Part model, mm, in its own coordinate system. Face numbers are marked on the shaded views. A direction names the side the tool comes from. Round coordinates to 2 decimals unless told otherwise and drop trailing zeros. Loops run counter-clockwise (first coordinate to the right, second up) from the corner with the lowest first, then second, coordinate; pieces in that order, holes last. Notation, with made-up numbers: (-18.75, 45) - (39.25, 45) arc R29 ccw to (39.25, 66) - close; hole circle Ø9 at (40, 28.5). An arc over 180 degrees is marked (long way). Put each result on its own line as item: value.
Autodesk Inventor part; units mm, degrees
ref_plane "YZ Plane" through (0, 0, 0) normal (1, 0, 0) x (0, 1, 0)
ref_plane "XZ Plane" through (0, 0, 0) normal (0, 1, 0) x (-1, 0, 0)
ref_plane "XY Plane" through (0, 0, 0) normal (0, 0, 1) x (1, 0, 0)
sketch "Sketch1" plane through (0, 0, 0) normal (0, 0, 1) x (1, 0, 0)
  line L0 (0, 0) -> (-38.1, 0)
  line L1 (-19.05, 0) -> (-19.05, -38.1)
  line L2 (-19.05, -38.1) -> (-38.1, -38.1)
  line L3 (-38.1, -38.1) -> (-38.1, 0)
  line L4 (-19.05, -38.1) -> (0, -38.1)
  line L5 (0, 0) -> (0, -38.1)
  dimension "d0" = 38.1
  dimension "d1" = 38.1
  dimension "d2" = 19.05
  dimension "d3" = 19.05
extrude "Plate1" add sketch "Sketch1" along normal blind 3.048
sketch "Sketch2" plane through (0, 0, 3.048) normal (0, 0, 1) x (1, 0, 0)
  line L0 (-38.1, 0) -> (0, 0)
  line L1 (0, -38.1) -> (-38.1, -38.1)
  line L2 (-19.05, 0) -> (-19.05, -19.05)
  circle A0 centre (-19.05, -19.05) radius 14.2875
  dimension "d7" = 19.05
  dimension "d8" = 28.575
extrude "Cut1" cut sketch "Sketch2" against normal blind 3.048
sketch "Sketch3" plane through (-38.1, -41.148, -3.048) normal (0, -1, 0) x (1, 0, 0)
  line L0 (38.1, 0) -> (0, 0)
  line L1 (0, 0) -> (0, -19.304)
  line L2 (0, -19.304) -> (38.1, -19.304)
  line L3 (38.1, -19.304) -> (38.1, 0)
edge flange "Flange1" height 25.4 angle 90 thickness 3.048 bend radius 3.048 thickness toward (0, -1, 0) relief straight relief width 3.048 relief depth 1.524 edges at (-19.05, -38.1, 0) wall of the first edge with corners at (0, -41.148, -3.048) (-38.1, -41.148, -3.048) (-38.1, -41.148, -22.352) (0, -41.148, -22.352)
bend "Bend1"
corner "Corner1"
sketch "Sketch5" plane through (-38.1, -41.148, -22.352) normal (0, 1, 0) x (1, 0, 0)
  line L0 (0, -19.304) -> (38.1, -19.304)
  line L1 (38.1, 0) -> (38.1, -19.304)
  line L2 (38.1, 0) -> (0, 0)
  line L3 (0, 0) -> (0, -19.304)
  point P0 (38.1, -22.352)
equation "\"d9\" = Thickness"
equation "\"d11\" = BendReliefWidth"
equation "\"d12\" = BendReliefDepth"
equation "\"d13\" = MinimumRemnant"
equation "\"d14\" = BendRadius"
equation "\"d17\" = BendRadius"
equation "\"d18\" = CornerReliefSize"
equation "\"d19\" = GapSize"
equation "\"d20\" = JacobiRadiusSize"
equation "\"BendRadius\" = Thickness"
equation "\"BendReliefWidth\" = Thickness"
equation "\"BendReliefDepth\" = 0.5 * Thickness"
equation "\"CornerReliefSize\" = 4 * Thickness"
equation "\"MinimumRemnant\" = 2 * Thickness"
equation "\"TransitionRadius\" = BendRadius"
equation "\"JacobiRadiusSize\" = Thickness"
equation "\"GapSize\" = Thickness"
equation "\"d4\" = BendRadius"
properties part number "arm assembly outer mount"
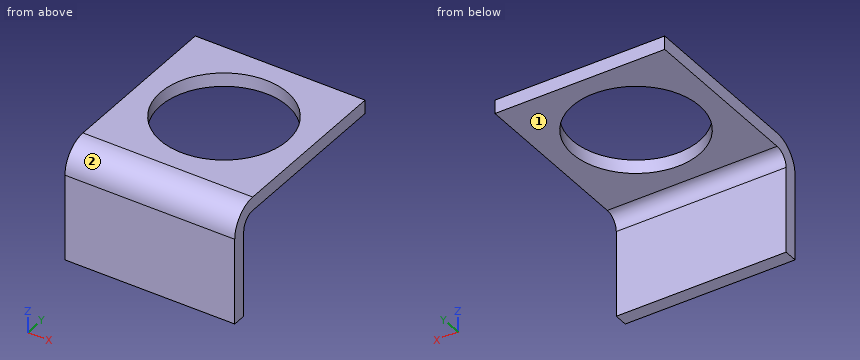
1. Band-saw the part on B-B (y = -19.05). List the corners of the cut face in (x, z), plus the area to 3 significant figures.
A:
outline: (-38.1, 0) - (-33.34, 0) - (-33.34, 3.05) - (-38.1, 3.05) - close; (-4.76, 0) - (0, 0) - (0, 3.05) - (-4.76, 3.05) - close
area: 29.0 mm²
2. Pin check, flat tip, straight feed: P1, Ø17, axis at x = -19.05, y = -19.05, coming from the -Z side. Stop position of the tip, or through.
A:
P1: passes through
3. Band-saw the part on D-D (x = -30.5). List the corners of the cut face in (y, z), plus the area to 3 significant figures.
A:
outline: (-44.2, -22.35) - (-41.15, -22.35) - (-41.15, -3.05) arc R3.05 cw to (-38.1, 0) - (-27.6, 0) - (-27.6, 3.05) - (-38.1, 3.05) arc R6.1 ccw to (-44.2, -3.05) - close; (-10.5, 0) - (0, 0) - (0, 3.05) - (-10.5, 3.05) - close
area: 145 mm²
4. Band-saw the part on A-A (x = -19.05). List the corners of the cut face in (y, z).
A:
outline: (-44.2, -22.35) - (-41.15, -22.35) - (-41.15, -3.05) arc R3.05 cw to (-38.1, 0) - (-33.34, 0) - (-33.34, 3.05) - (-38.1, 3.05) arc R6.1 ccw to (-44.2, -3.05) - close; (-4.76, 0) - (0, 0) - (0, 3.05) - (-4.76, 3.05) - close
5. Band-saw the part on C-C (z = -13.25). List the corners of the cut face in (x, y).
A:
outline: (-38.1, -44.2) - (0, -44.2) - (0, -41.15) - (-38.1, -41.15) - close
6. Tool access for the marked faces 1 and 2: list every direction of +Z, -Z, +X, -X, +Y, -Y with a clear straight run to the whole face (end or side of a thin tool).
A:
face 1: -Z, +X, -X, +Y
face 2: +Z, +X, -X, -Y
7. Probe line 1 along X through (y, z) = (-19.05, 0.95); line 2 along Y through (x, z) = (-1.5, -6.25); line 3 along Z through (x, y) = (-5, -10). List the from-to ranges inside material, lowest first. Write a range as [from, to].
A:
line 1: x = [-38.1, -33.34], [-4.76, 0]
line 2: y = [-44.2, -41.15]
line 3: z = [0, 3.05]
